Can you work these out from the model? Positions are in its coordinate system, mm. Coordinates: 2 decimals unless noted, no trailing zeros. Loops run counter-clockwise (first coordinate to the right, second up) from the corner with the lowest first, then second, coordinate; pieces in that order, holes last.
```python
from build123d import *

# Parameters (mm, degrees)
SALIENTE_EXTRUIR1_DEPTH = 1.5
CROQUIS2_R              = 1.5
CORTAR_EXTRUIR1_DEPTH   = 1.5


with BuildPart() as part:
    # Croquis1 → Saliente-Extruir1 (new body)
    with BuildSketch(Plane(origin=(0, 0, 0), x_dir=(1, 0, 0), z_dir=(0, 1, 0))):
        with BuildLine():
            ThreePointArc((23.270329614, 12), (29.541594579, 15.310243942), (34.860679775, 20))
            ThreePointArc((34.860679775, 20), (42.5, 40), (34.860679775, 60))
            ThreePointArc((34.860679775, 60), (29.541594579, 64.689756058), (23.270329614, 68))
            ThreePointArc((23.270329614, 68), (17.977225575, 69.495762408), (12.5, 70))
            Line((12.5, 70), (12.5, 10))
            ThreePointArc((12.5, 10), (17.977225575, 10.504237592), (23.270329614, 12))
        make_face()
        Polygon((-40, 0), (-40, -40), (40, -40), (40, 0), (34.860679775, 0), (23.270329614, 0), (12.5, 0), (12.5, 10), (12.5, 70), (12.5, 80), (23.270329614, 80), (34.860679775, 80), (40, 80), (40, 120), (-40, 120), (-40, 80), (-34.860679775, 80), (-23.270329614, 80), (-12.5, 80), (-12.5, 70), (-12.5, 40), (-12.5, 10), (-12.5, 0), (-23.270329614, 0), (-34.860679775, 0), align=None)
        with BuildLine():
            ThreePointArc((-34.860679775, 60), (-42.5, 40), (-34.860679775, 20))
            ThreePointArc((-34.860679775, 20), (-29.541594579, 15.310243942), (-23.270329614, 12))
            ThreePointArc((-23.270329614, 12), (-17.977225575, 10.504237592), (-12.5, 10))
            Line((-12.5, 10), (-12.5, 40))
            Line((-12.5, 40), (-12.5, 70))
            ThreePointArc((-12.5, 70), (-17.977225575, 69.495762408), (-23.270329614, 68))
            ThreePointArc((-23.270329614, 68), (-29.541594579, 64.689756058), (-34.860679775, 60))
        make_face()
        with BuildLine():
            Line((23.270329614, 0), (34.860679775, 0))
            Line((34.860679775, 0), (34.860679775, 20))
            ThreePointArc((34.860679775, 20), (29.541594579, 15.310243942), (23.270329614, 12))
            Line((23.270329614, 12), (23.270329614, 0))
        make_face()
        with BuildLine():
            ThreePointArc((23.270329614, 68), (29.541594579, 64.689756058), (34.860679775, 60))
            Line((34.860679775, 60), (34.860679775, 80))
            Line((34.860679775, 80), (23.270329614, 80))
            Line((23.270329614, 80), (23.270329614, 68))
        make_face()
        with BuildLine():
            Line((-34.860679775, 80), (-34.860679775, 60))
            ThreePointArc((-34.860679775, 60), (-29.541594579, 64.689756058), (-23.270329614, 68))
            Line((-23.270329614, 68), (-23.270329614, 80))
            Line((-23.270329614, 80), (-34.860679775, 80))
        make_face()
        with BuildLine():
            Line((-34.860679775, 20), (-34.860679775, 0))
            Line((-34.860679775, 0), (-23.270329614, 0))
            Line((-23.270329614, 0), (-23.270329614, 12))
            ThreePointArc((-23.270329614, 12), (-29.541594579, 15.310243942), (-34.860679775, 20))
        make_face()
    extrude(amount=SALIENTE_EXTRUIR1_DEPTH)

    # Croquis2 → Cortar-Extruir1 (cut)
    with BuildSketch(Plane(origin=(0, 1.5, 0), x_dir=(1, 0, 0), z_dir=(0, 1, 0))):
        with Locations(Location((32, -20, 0), (0, 0, 270))):
            Circle(CROQUIS2_R)
        with Locations(Location((29.071067812, -27.071067812, 0), (0, 0, 270))):
            Circle(CROQUIS2_R)
        with Locations(Location((22, -30, 0), (0, 0, 270))):
            Circle(CROQUIS2_R)
        with Locations(Location((14.928932188, -27.071067812, 0), (0, 0, 270))):
            Circle(CROQUIS2_R)
        with Locations(Location((12, -20, 0), (0, 0, 270))):
            Circle(CROQUIS2_R)
        with Locations(Location((14.928932188, -12.928932188, 0), (0, 0, 270))):
            Circle(CROQUIS2_R)
        with Locations(Location((22, -10, 0), (0, 0, 270))):
            Circle(CROQUIS2_R)
        with Locations(Location((29.071067812, -12.928932188, 0), (0, 0, 270))):
            Circle(CROQUIS2_R)
        with Locations(Location((-29.071067812, -12.928932188, 0), (0, 0, 90))):
            Circle(CROQUIS2_R)
        with Locations(Location((-22, -10, 0), (0, 0, 90))):
            Circle(CROQUIS2_R)
        with Locations(Location((-14.928932188, -12.928932188, 0), (0, 0, 90))):
            Circle(CROQUIS2_R)
        with Locations(Location((-12, -20, 0), (0, 0, 90))):
            Circle(CROQUIS2_R)
        with Locations(Location((-14.928932188, -27.071067812, 0), (0, 0, 90))):
            Circle(CROQUIS2_R)
        with Locations(Location((-22, -30, 0), (0, 0, 90))):
            Circle(CROQUIS2_R)
        with Locations(Location((-29.071067812, -27.071067812, 0), (0, 0, 90))):
            Circle(CROQUIS2_R)
        with Locations(Location((-32, -20, 0), (0, 0, 90))):
            Circle(CROQUIS2_R)
        with Locations(Location((-32, 100, 0), (0, 0, 270))):
            Circle(CROQUIS2_R)
        with Locations(Location((-29.071067812, 107.071067812, 0), (0, 0, 270))):
            Circle(CROQUIS2_R)
        with Locations(Location((-22, 110, 0), (0, 0, 270))):
            Circle(CROQUIS2_R)
        with Locations(Location((-14.928932188, 107.071067812, 0), (0, 0, 270))):
            Circle(CROQUIS2_R)
        with Locations(Location((-12, 100, 0), (0, 0, 270))):
            Circle(CROQUIS2_R)
        with Locations(Location((-14.928932188, 92.928932188, 0), (0, 0, 270))):
            Circle(CROQUIS2_R)
        with Locations(Location((-22, 90, 0), (0, 0, 270))):
            Circle(CROQUIS2_R)
        with Locations(Location((-29.071067812, 92.928932188, 0), (0, 0, 270))):
            Circle(CROQUIS2_R)
        with Locations(Location((29.071067812, 92.928932188, 0), (0, 0, 90))):
            Circle(CROQUIS2_R)
        with Locations(Location((22, 90, 0), (0, 0, 90))):
            Circle(CROQUIS2_R)
        with Locations(Location((14.928932188, 92.928932188, 0), (0, 0, 90))):
            Circle(CROQUIS2_R)
        with Locations(Location((12, 100, 0), (0, 0, 90))):
            Circle(CROQUIS2_R)
        with Locations(Location((14.928932188, 107.071067812, 0), (0, 0, 90))):
            Circle(CROQUIS2_R)
        with Locations(Location((22, 110, 0), (0, 0, 90))):
            Circle(CROQUIS2_R)
        with Locations(Location((29.071067812, 107.071067812, 0), (0, 0, 90))):
            Circle(CROQUIS2_R)
        with Locations(Location((32, 100, 0), (0, 0, 90))):
            Circle(CROQUIS2_R)
    extrude(amount=-CORTAR_EXTRUIR1_DEPTH, mode=Mode.SUBTRACT)


solid = part.part
```
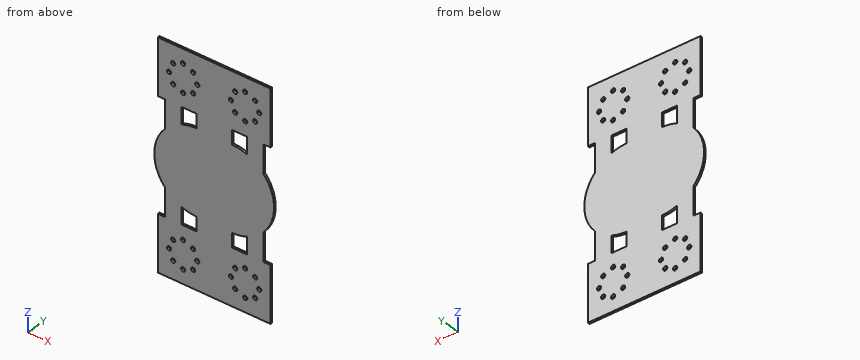
Item 1: Suppose I cut it at C-C, the plane z = 23.5. Please give me the cut outline in (x, y).
Results are:
outline: (-40, 0) - (40, 0) - (40, 1.5) - (-40, 1.5) - close
Item 2: I'm going to push a flat-ended pin straight in: P1, Ø2.5, axis at x = 14.93, z = 12.93, coming from the -Y side. Where does the tip first touch, or does it pass through?
Results are:
P1: passes through
Item 3: Suppose I cut it at B-B, the plane y = 0.8. Count the separate pieces of the cut face and the enclosed holes in it, plus the area to 3 significant figures.
Results are:
separate pieces: 1
enclosed holes: 36
area: 11,700 mm2
Item 4: Suppose I cut it at A-A, the plane z = -73. Please give me the cut outline in (x, y).
Results are:
outline: (-34.86, 0) - (-23.27, 0) - (-23.27, 1.5) - (-34.86, 1.5) - close; (-12.5, 0) - (12.5, 0) - (12.5, 1.5) - (-12.5, 1.5) - close; (23.27, 0) - (34.86, 0) - (34.86, 1.5) - (23.27, 1.5) - close
Item 5: I need wall thicknesses on line 1 along X through (y, z) = (1, -73); line 2 along X through (y, z) = (0.95, -90); line 3 along X through (y, z) = (0.65, 20). Which ranges of each line are inside material? Lowest first, please.
Results are:
line 1: x = -34.86 to -23.27, -12.5 to 12.5, 23.27 to 34.86
line 2: x = -40 to -23.5, -20.5 to 20.5, 23.5 to 40
line 3: x = -40 to -33.5, -30.5 to -13.5, -10.5 to 10.5, 13.5 to 30.5, 33.5 to 40
